from build123d import *

# Parameters (mm, degrees)
SKETCH_1_R          = 7.5
EXTRUDE_1_DEPTH     = 30
SKETCH_2_W          = 2
SKETCH_2_H          = 20
CUT_EXTRUDE_1_DEPTH = 10


with BuildPart() as part:
    # 草图1 → 凸台-拉伸1 (new body, symmetric)
    with BuildSketch(Plane.XY):
        Circle(SKETCH_1_R)
    extrude(amount=EXTRUDE_1_DEPTH, both=True)

    # 草图2 → 切除-拉伸1 (cut, symmetric)
    with BuildSketch(Plane(origin=(0, 0, 0), x_dir=(1, 0, 0), z_dir=(0, 1, 0))):
        with Locations((-7.5, 0)):
            Rectangle(SKETCH_2_W, SKETCH_2_H)
        with Locations((7.5, 0)):
            Rectangle(SKETCH_2_W, SKETCH_2_H)
    extrude(amount=CUT_EXTRUDE_1_DEPTH, both=True, mode=Mode.SUBTRACT)

    # 草图5 → M6 螺纹孔1 (revolve, cut)
    with BuildSketch(Plane(origin=(0, 0, -30), x_dir=(0, 1, 0), z_dir=(1, 0, 0))):
        Polygon((0, 0), (0, 16.502151548), (2.5, 15), (2.5, 0), align=None)
    hole_wizard_m6_1 = revolve(axis=Axis((0, 0, -36.35), (0, 0, 1)), mode=Mode.SUBTRACT)

    # 镜向1: M6 螺纹孔1 across plane
    add(hole_wizard_m6_1.mirror(Plane.XY), mode=Mode.SUBTRACT)


solid = part.part
The model under review builds one solid part; all positions refer to its coordinate system, in mm. A direction names the side the tool comes from. Give positions to 0.01 mm unless a question says otherwise; leave off trailing zeros. Loops run counter-clockwise (first coordinate to the right, second up) from the corner with the lowest first, then second, coordinate; pieces in that order, holes last. Notation, with made-up numbers: (37, -35.5) -> (65, -35.5) arc R24 ccw to (65, -20.5) -> close; hole circle Ø4 at (-12.75, 50). An arc over 180 degrees is marked (long way). Put each result on its own line as item: value. Start each with the question number.
1. Mouldability with a two-part tool opening along Y and no side actions: class faces 1 (the face through (-5.5, 5.1, 0.4)), 2 (the face through (2.44, -0.54, -22.6)), 3 (the face through (-7, 0, -10)) as released by +Y, released by -Y, zero draft, split by the parting line, or undercut.
2. We need section B-B on x = 5.25. State the section outline as (y, z) points, then the cut area to 3 significant figures.
3. Wall thickness on probe 1 along Y at (x, z) = (0, 22); probe 2 along Y at (x, z) = (-0.25, -7): over which ranges is each line inside the solid? List them lowest first.
4. Clearance check with flat-ended pins moving along their axes: P1, Ø8, axis at y = 4.5, z = -18, coming from the +X side; P2, Ø2, axis at x = 2.5, z = -21.5, coming from the +Y side; P3, Ø6, axis at y = 0.5, z = -4.5, coming from the -X side. State where each tip first meets the part, or that it passes through.
5. For faces 4 (the face through (-7, 0, 10)), 5 (the face through (2.44, -0.54, 22.6)), 6 (the face through (7, 0, -10)), list the 3-axis set-ups (+Z, -Z, +X, -X, +Y, -Y) from which the entire face can be reached by the end or side of a thin tool; tool diameter is ignored.
6. We need section A-A on y = -6. State the section outline as (x, z) points.
Determined:
1. face 1: split by the parting line
1. face 2: undercut
1. face 3: zero draft
2. outline: (-5.36, -30) -> (5.36, -30) -> (5.36, 30) -> (-5.36, 30) -> close
2. area: 643 mm^2
3. probe 1: -7.5 to -2.5, 2.5 to 7.5
3. probe 2: -7.5 to 7.5
4. P1: x = 7.48
4. P2: y = 7.35
4. P3: x = -6.5
5. face 4: -X, +Y, -Y
5. face 5: +Z
5. face 6: +X, +Y, -Y
6. outline: (-4.5, -30) -> (4.5, -30) -> (4.5, 30) -> (-4.5, 30) -> close
